Can you work these out from the model? Positions are in its coordinate system, mm. Coordinates: 2 decimals unless noted, no trailing zeros. Write each loop counter-clockwise with the first axis right and the second up, starting at its lowest first coordinate (ties: lowest second). Pieces come first, ordered by that corner, then holes. Notation, with made-up numbers: (-2, -37) -> (51, -37) arc R23 cw to (51, -26) -> close; hole circle Ø11 at (40.25, -31.75). An arc over 180 degrees is marked (long way). Use one line per item in the form item = value.
```python
from build123d import *

# Parameters (mm, degrees)
F1_DEPTH = 2800
F3_W     = 662.5
F3_H     = 450
F4_DEPTH = 247


with BuildPart() as f1:
    # F0 (on Front) → F1 (new body)
    with BuildSketch(Plane.XZ):
        Polygon((300, 0), (0, 0), (0, -450), align=None)
    extrude(amount=F1_DEPTH)

    # F3 (on face) → F4 (cut)
    with BuildSketch(Plane(origin=(172.36, 0, -80.372788), x_dir=(0, -1, 0), z_dir=(-0.906308, 0, 0.422618))):
        with Locations((2438.75, -152.838504)):
            Rectangle(F3_W, F3_H)
        with Locations((1746.25, -152.838504)):
            Rectangle(F3_W, F3_H)
        with Locations((1053.75, -152.838504)):
            Rectangle(F3_W, F3_H)
        with Locations((361.25, -152.838504)):
            Rectangle(F3_W, F3_H)
    extrude(amount=-F4_DEPTH, mode=Mode.SUBTRACT)


solid = f1.part
```
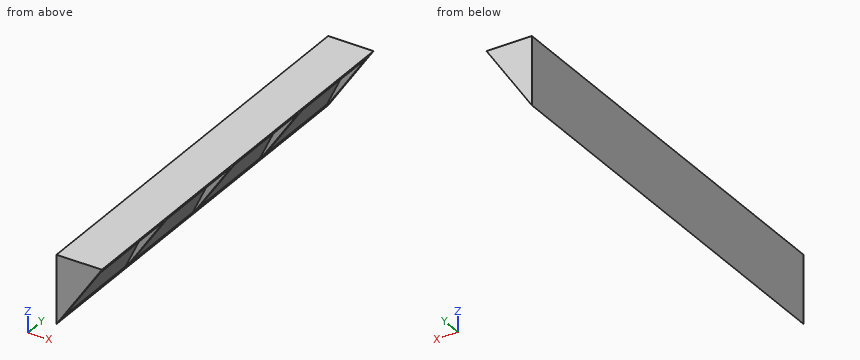
Q1. Will this pin go through, and if not, where does the flat tip stop? pin 1 (6 mm diameter, centred on y = -893.5, z = -333.5, fed in from +X).
Return value:
pin_1 = 55.72
Q2. Suppose I cut it at B-B (z = -325.5). Write out the boundary of the cut face in (x, y), then the cut area to 3 significant figures.
Return value:
outline = (0, -2800) -> (83, -2800) -> (83, -2770) -> (58.06, -2770) -> (58.06, -2107.5) -> (83, -2107.5) -> (83, -2077.5) -> (58.06, -2077.5) -> (58.06, -1415) -> (83, -1415) -> (83, -1385) -> (58.06, -1385) -> (58.06, -722.5) -> (83, -722.5) -> (83, -692.5) -> (58.06, -692.5) -> (58.06, -30) -> (83, -30) -> (83, 0) -> (0, 0) -> close
area = 166,000 mm2
Q3. Suppose I cut it at A-A (y = -1438.5). Write out the boundary of the cut face in (x, z), then the cut area to 3 significant figures.
Return value:
outline = (0, -450) -> (16.83, -424.75) -> (12.68, -422.81) -> (202.86, -14.97) -> (269.35, -45.98) -> (300, 0) -> (0, 0) -> close
area = 50,000 mm2
Q4. If I drill on line 1 (Z direction, x = 235, y = -1456.5); line 2 (X direction, y = -643.5, z = -25); line 3 (Z direction, x = 103, y = -2426.5), over which ranges is the centre line in solid material (lowest first)? Write a range as from..to.
Return value:
line_1 = -29.96..0
line_2 = 0..198.18, 224.36..283.33
line_3 = -229.12..0
Q5. Suppose I cut it at C-C (x = 45). Write out the boundary of the cut face in (y, z).
Return value:
outline = (-2800, -382.5) -> (-2770, -382.5) -> (-2770, -353.5) -> (-2107.5, -353.5) -> (-2107.5, -382.5) -> (-2077.5, -382.5) -> (-2077.5, -353.5) -> (-1415, -353.5) -> (-1415, -382.5) -> (-1385, -382.5) -> (-1385, -353.5) -> (-722.5, -353.5) -> (-722.5, -382.5) -> (-692.5, -382.5) -> (-692.5, -353.5) -> (-30, -353.5) -> (-30, -382.5) -> (0, -382.5) -> (0, 0) -> (-2800, 0) -> close
